```python
from build123d import *

# Parameters (mm, degrees)
EXTRUDE_1_DEPTH     = 6
EXTRUDE_2_DEPTH     = 6
SKETCH_3_R          = 1.55
CUT_EXTRUDE_1_DEPTH = 6


with BuildPart() as part:
    # Эскиз1 → Бобышка-Вытянуть1 (new body)
    with BuildSketch(Plane.XY):
        Polygon((-114.323496858, 125.813994573), (-171.575189585, 135.638663443), (-164.719145048, 155.026651824), (-114.323496858, 146.378513535), align=None)
    extrude(amount=EXTRUDE_1_DEPTH)

    # Эскиз2 → Бобышка-Вытянуть2 (add)
    with BuildSketch(Plane(origin=(0, 0, 0), x_dir=(-1, 0, 0), z_dir=(0, 0, -1))):
        Polygon((146.738238306, 131.376521829), (139.160448137, 130.076136187), (139.160448137, 150.64065515), (139.882193768, 150.76451021), align=None)
    extrude(amount=EXTRUDE_2_DEPTH)

    # Эскиз3 → Вырез-Вытянуть1 (cut)
    with BuildSketch(Plane(origin=(0, 0, 0), x_dir=(-1, 0, 0), z_dir=(0, 0, -1))):
        with Locations((126.643413167, 138.210411601)):
            Circle(SKETCH_3_R)
        with Locations((155.827251007, 143.218500087)):
            Circle(SKETCH_3_R)
    extrude(amount=-CUT_EXTRUDE_1_DEPTH, mode=Mode.SUBTRACT)


solid = part.part
```
Check sheet for the modelled part. Datum: model origin and axes. Units: mm. A direction names the side the tool comes from. Coordinates: 2 decimals unless noted, no trailing zeros. Order: outer loops, then holes, each group sorted by start corner. A loop starts at its lowest first (then second) coordinate and runs counter-clockwise, first axis right, second up. Notation, with made-up numbers: M 32.5,-12 L 83.5,-12 A32 ccw 83.5,25 Z; hole C 88,61.5 d5. An arc over 180 degrees is marked long. One line per question, with ' | ' between items. Start each with the question number.
Item 1: Gauge pin test, flat ends, axial feed: P1, Ø12, axis at x = -160.5, y = 141.5, coming from the -Z side; P2, Ø12, axis at x = -157, y = 142.5, coming from the +Z side; P3, Ø5, axis at y = 139, z = -4, coming from the -X side; P4, Ø1.9, axis at x = -155.83, y = 143.22, coming from the -Z side. Record the tip position at first contact, or that the pin passes through.
Item 2: Sectioned sample at A-A on x = -156. Record the cut outline in (y, z).
Item 3: Sectioned sample at B-B on z = 3.5. Record the cut outline in (x, y), and give its area (3 significant figures).
Item 4: Sectioned sample at C-C on y = 134.25. Record the cut outline in (x, z).
Item 5: Material ranges on line 1 (Z direction, x = -136.5, y = 132.75); line 2 (X direction, y = 144.5, z = 2.75); line 3 (Y direction, x = -125.5, z = 5.5), recorded low to high.
Item 6: Sectioned sample at D-D on z = -4.25. Record the cut outline in (x, y).
Item 7: Access from +Z, -Z, +X, -X, +Y, -Y to the whole of each face (thin tool, end or side, straight path). Record for faces 4 (the flat face through (-156, 141, 0)), 5 (the flat face through (-168.195, 145.197, 2.958)), 6 (the flat face through (-127, 136, 0)).
Item 8: Mould release check, pull along Y, two halves, no side actions. Record for faces 1 (the cylindrical face through (-154.28, 143.29, 2.96)), 2 (the flat face through (-139.16, 140, -3)), 3 (the flat face through (-143.26, 141.21, -2.96)): pulls with the +Y half, pulls with the -Y half, needs draft (parallel to the pull), parting line crosses it, or undercut.
Answer below:
1) P1: stops at z = 0 | P2: stops at z = 6 | P3: stops at x = -144.93 | P4: passes through
2) outline: M 132.97,0 L 141.68,0 L 141.68,6 L 132.97,6 Z; M 144.76,0 L 153.53,0 L 153.53,6 L 144.76,6 Z
3) outline: M -171.58,135.64 L -114.32,125.81 L -114.32,146.38 L -164.72,155.03 Z; hole C -155.83,143.22 d3.1; hole C -126.64,138.21 d3.1 | area: 1,090 mm^2
4) outline: M -163.48,0 L -145.72,0 L -145.72,-6 L -139.16,-6 L -139.16,0 L -114.32,0 L -114.32,6 L -163.48,6 Z
5) line 1: z = 0 to 6 | line 2: x = -168.44 to -156.7, -154.96 to -114.32 | line 3: y = 127.73 to 137.16, 139.26 to 148.3
6) outline: M -146.74,131.38 L -139.16,130.08 L -139.16,150.64 L -139.88,150.76 Z
7) face 4: -Z, -X, +Y | face 5: +Z, -Z, -X, +Y | face 6: -Z, +X, +Y, -Y
8) face 1: undercut | face 2: needs draft | face 3: pulls with the +Y half
